Print and shaded views of the part. All mm, measured from the part's lowest x, y and z. Round coordinates to 2 decimals unless told otherwise and drop trailing zeros. Write each loop counter-clockwise with the first axis right and the second up, starting at its lowest first coordinate (ties: lowest second). Pieces come first, ordered by that corner, then holes. Notation, with made-up numbers: (26.5, 62) - (47.5, 62) arc R28 cw to (47.5, 85) - close; hole circle Ø8 at (39, 14.5). An arc over 180 degrees is marked (long way). Put each result on its own line as item: value. Start each with the question number.
Item 1: Cut at A-A (y = 128.5). Give the cut face in (x, z), and give its area (3 significant figures).
Item 2: Cut at C-C (z = 1.5). Give the cut face in (x, y), and give its area (3 significant figures).
Item 3: Pin check, flat tip, straight feed: pin 1 Ø3 at (x, y) = (39.5, 131) entering from +Z. Stop position of the tip, or through.
Item 4: Cut at B-B (x = 9.5). Give the cut face in (y, z), and give its area (3 significant figures).
Item 5: Drill centre lines: line 1 (X direction, y = 99.5, z = 5.5); line 2 (Y direction, x = 40.5, z = 5.5); line 3 (X direction, y = 91, z = 5.75). Where is each one in solid material? Low to high. Write a range as from..to.
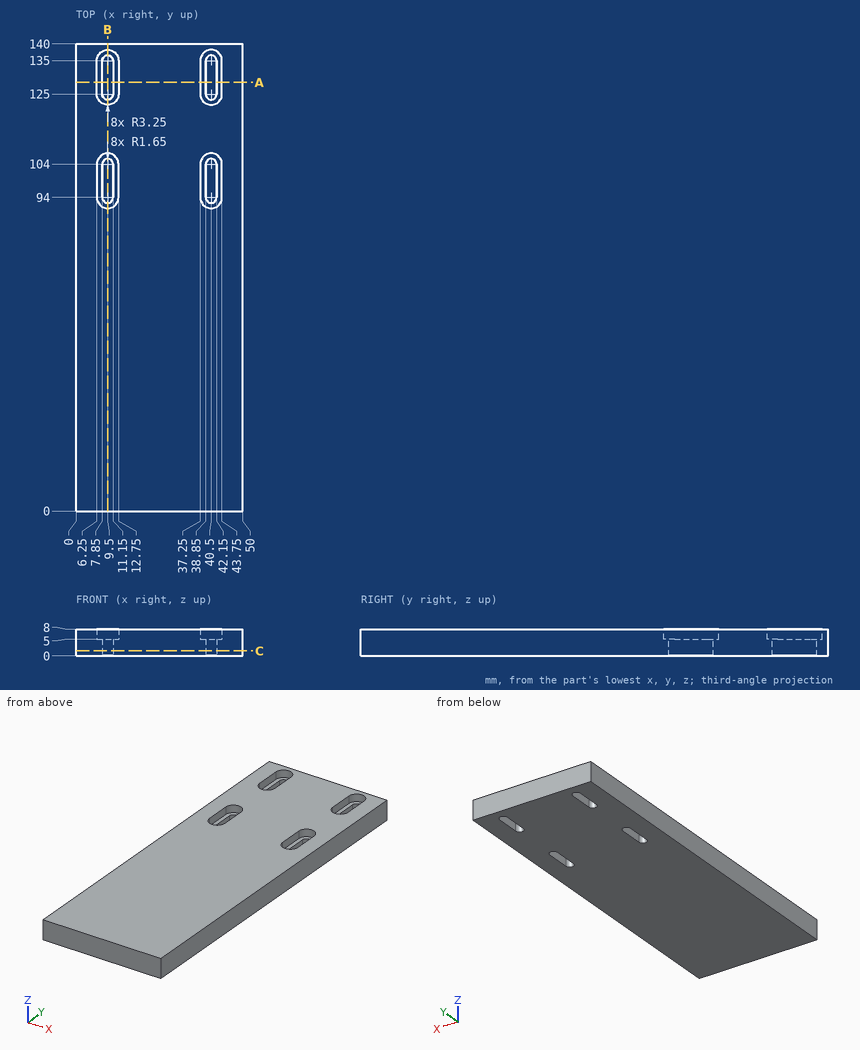
Output values:
1. outline: (0, 0) - (7.85, 0) - (7.85, 5) - (6.25, 5) - (6.25, 8) - (0, 8) - close; (11.15, 0) - (38.85, 0) - (38.85, 5) - (37.25, 5) - (37.25, 8) - (12.75, 8) - (12.75, 5) - (11.15, 5) - close; (42.15, 0) - (50, 0) - (50, 8) - (43.75, 8) - (43.75, 5) - (42.15, 5) - close
1. area: 328 mm2
2. outline: (0, 0) - (50, 0) - (50, 140) - (0, 140) - close; hole (7.85, 94) arc R1.65 ccw to (11.15, 94) - (11.15, 104) arc R1.65 ccw to (7.85, 104) - close; hole (7.85, 125) arc R1.65 ccw to (11.15, 125) - (11.15, 135) arc R1.65 ccw to (7.85, 135) - close; hole (38.85, 94) arc R1.65 ccw to (42.15, 94) - (42.15, 104) arc R1.65 ccw to (38.85, 104) - close; hole (38.85, 125) arc R1.65 ccw to (42.15, 125) - (42.15, 135) arc R1.65 ccw to (38.85, 135) - close
2. area: 6,830 mm2
3. pin 1: z = 5
4. outline: (0, 0) - (92.35, 0) - (92.35, 5) - (90.75, 5) - (90.75, 8) - (0, 8) - close; (105.65, 0) - (123.35, 0) - (123.35, 5) - (121.75, 5) - (121.75, 8) - (107.25, 8) - (107.25, 5) - (105.65, 5) - close; (136.65, 0) - (140, 0) - (140, 8) - (138.25, 8) - (138.25, 5) - (136.65, 5) - close
4. area: 888 mm2
5. line 1: 0..6.25, 12.75..37.25, 43.75..50
5. line 2: 0..90.75, 107.25..121.75, 138.25..140
5. line 3: 0..8.25, 10.75..39.25, 41.75..50
